Model file for the job. Use its own axes, mm. Face numbers are marked on the shaded views. A direction names the side the tool comes from. Coordinates: 2 decimals unless noted, no trailing zeros. Write each loop counter-clockwise with the first axis right and the second up, starting at its lowest first coordinate (ties: lowest second). Pieces come first, ordered by that corner, then holes. Notation, with made-up numbers: (78.25, 25.25) - (122.25, 25.25) arc R30 cw to (122.25, 53.25) - close; hole circle Ø2 at (54.25, 14.5). An arc over 180 degrees is marked (long way). Put each result on its own line as item: value. Start each with the question number.
1. Saw through at A-A, the plane y = -38.5. Write the cut outline in (x, z).
2. Saw through at C-C, the plane x = -27.5. Write the cut outline in (y, z), plus the area to 3 significant figures.
3. Drill centre lines: L1, parallel to Y at x = -14.5, z = 4.5; L2, parallel to X at y = -35.75, z = 4.5; L3, parallel to X at y = -43.25, z = 4. Where is each one in solid material? Low to high. Write a range as from..to.
4. Drop flat-ended pins along their axis: P1, Ø2, axis at y = -47, z = 6, coming from the -X side; P2, Ø1.5, axis at y = -39, z = 1, coming from the +X side. Give the stop position or say it passes through.
5. Pull direction X, two halves, no side cores. Call the marked faces 4, 5, 6 and 7: released by +X, released by -X, zero draft, split by the parting line, or undercut.
6. Which spindle directions (+Z, -Z, +X, -X, +Y, -Y) get a long thin tool onto all of the face, cutting with end or side? Do the marked faces 1, 2 and 3. Say none if no direction does.
7. Saw through at D-D, the plane z = 6. Write the cut outline in (x, y), plus the area to 3 significant figures.
8. Saw through at B-B, the plane z = 3. Write the cut outline in (x, y), plus the area to 3 significant figures.
```python
from build123d import *

# Parameters (mm, degrees)
F1_DEPTH     = 7
F2_T1_DEPTH  = 32
F2_T3_DEPTH  = 40
F2_T5_DEPTH  = 22
F2_T7_DEPTH  = 11
F2_T10_ANGLE = 90
F2_T12_ANGLE = 90
F2_T14_ANGLE = 90
F2_T16_ANGLE = 90
F2_T18_ANGLE = 90
F2_T20_ANGLE = 90
F2_T22_ANGLE = 90
F2_T24_ANGLE = 90


# Not quite as in the source:
# - a fillet or chamfer that OpenCascade refuses, or shapes differently, is made with other operations: its cross-section is extruded or revolved along the edge and cut away or added


with BuildPart() as f1:
    # F0 (on Top) → F1 (new body)
    with BuildSketch(Plane.XY):
        with BuildLine():
            Line((-4.4512270018, -28.9949133558), (-54.4512270018, -28.9949133558))
            Line((-54.4512270018, -28.9949133558), (-54.4512270018, -45.9949133558))
            ThreePointArc((-54.4512270018, -45.9949133558), (-52.9867609078, -49.5304472618), (-49.4512270018, -50.9949133558))
            Line((-49.4512270018, -50.9949133558), (-9.4512270018, -50.9949133558))
            ThreePointArc((-9.4512270018, -50.9949133558), (-5.9156930959, -49.5304472618), (-4.4512270018, -45.9949133558))
            Line((-4.4512270018, -45.9949133558), (-4.4512270018, -28.9949133558))
        make_face()
        with BuildLine():
            Line((-50.4512270018, -42.9949133558), (-50.4512270018, -31.9949133558))
            Line((-50.4512270018, -31.9949133558), (-8.4512270018, -31.9949133558))
            Line((-8.4512270018, -31.9949133558), (-8.4512270018, -42.9949133558))
            ThreePointArc((-8.4512270018, -42.9949133558), (-9.9156930959, -46.5304472618), (-13.4512270018, -47.9949133558))
            Line((-13.4512270018, -47.9949133558), (-45.4512270018, -47.9949133558))
            ThreePointArc((-45.4512270018, -47.9949133558), (-48.9867609078, -46.5304472618), (-50.4512270018, -42.9949133558))
        make_face(mode=Mode.SUBTRACT)
    extrude(amount=F1_DEPTH)

    # F2: fillet of radius 2 on 4 edges, made by hand

    # F2_s2 → F2_t1 (cut)
    with BuildSketch(Plane.YZ.offset(-45.4512270018)):
        with BuildLine():
            ThreePointArc((-47.9949133558, 5), (-48.5806997934, 6.4142135624), (-49.9949133558, 7))
            Line((-49.9949133558, 7), (-47.9949133558, 7))
            Line((-47.9949133558, 7), (-47.9949133558, 5))
        make_face()
        with BuildLine():
            ThreePointArc((-47.9949133558, 2), (-48.5806997934, 0.5857864376), (-49.9949133558, 0))
            Line((-49.9949133558, 0), (-47.9949133558, 0))
            Line((-47.9949133558, 0), (-47.9949133558, 2))
        make_face()
    extrude(amount=F2_T1_DEPTH, mode=Mode.SUBTRACT)

    # F2_s4 → F2_t3 (cut)
    with BuildSketch(Plane.YZ.offset(-49.4512270018)):
        with BuildLine():
            ThreePointArc((-50.9949133558, 5), (-50.4091269182, 6.4142135624), (-48.9949133558, 7))
            Line((-48.9949133558, 7), (-50.9949133558, 7))
            Line((-50.9949133558, 7), (-50.9949133558, 5))
        make_face()
        with BuildLine():
            ThreePointArc((-50.9949133558, 2), (-50.4091269182, 0.5857864376), (-48.9949133558, 0))
            Line((-48.9949133558, 0), (-50.9949133558, 0))
            Line((-50.9949133558, 0), (-50.9949133558, 2))
        make_face()
    extrude(amount=F2_T3_DEPTH, mode=Mode.SUBTRACT)

    # F2_s6 → F2_t5 (cut)
    with BuildSketch(Plane.XZ.offset(23.9949133558)):
        with BuildLine():
            ThreePointArc((-54.4512270018, 2), (-53.8654405642, 0.5857864376), (-52.4512270018, 0))
            Line((-52.4512270018, 0), (-54.4512270018, 0))
            Line((-54.4512270018, 0), (-54.4512270018, 2))
        make_face()
        with BuildLine():
            ThreePointArc((-4.4512270018, 2), (-5.0370134395, 0.5857864376), (-6.4512270018, 0))
            Line((-6.4512270018, 0), (-4.4512270018, 0))
            Line((-4.4512270018, 0), (-4.4512270018, 2))
        make_face()
        with BuildLine():
            ThreePointArc((-4.4512270018, 5), (-5.0370134395, 6.4142135624), (-6.4512270018, 7))
            Line((-6.4512270018, 7), (-4.4512270018, 7))
            Line((-4.4512270018, 7), (-4.4512270018, 5))
        make_face()
        with BuildLine():
            ThreePointArc((-54.4512270018, 5), (-53.8654405642, 6.4142135624), (-52.4512270018, 7))
            Line((-52.4512270018, 7), (-54.4512270018, 7))
            Line((-54.4512270018, 7), (-54.4512270018, 5))
        make_face()
    extrude(amount=F2_T5_DEPTH, mode=Mode.SUBTRACT)

    # F2_s8 → F2_t7 (cut)
    with BuildSketch(Plane.XZ.offset(31.9949133558)):
        with BuildLine():
            ThreePointArc((-50.4512270018, 2), (-51.0370134395, 0.5857864376), (-52.4512270018, 0))
            Line((-52.4512270018, 0), (-50.4512270018, 0))
            Line((-50.4512270018, 0), (-50.4512270018, 2))
        make_face()
        with BuildLine():
            ThreePointArc((-8.4512270018, 2), (-7.8654405642, 0.5857864376), (-6.4512270018, 0))
            Line((-6.4512270018, 0), (-8.4512270018, 0))
            Line((-8.4512270018, 0), (-8.4512270018, 2))
        make_face()
        with BuildLine():
            ThreePointArc((-50.4512270018, 5), (-51.0370134395, 6.4142135624), (-52.4512270018, 7))
            Line((-52.4512270018, 7), (-50.4512270018, 7))
            Line((-50.4512270018, 7), (-50.4512270018, 5))
        make_face()
        with BuildLine():
            ThreePointArc((-8.4512270018, 5), (-7.8654405642, 6.4142135624), (-6.4512270018, 7))
            Line((-6.4512270018, 7), (-8.4512270018, 7))
            Line((-8.4512270018, 7), (-8.4512270018, 5))
        make_face()
    extrude(amount=F2_T7_DEPTH, mode=Mode.SUBTRACT)

    # F2_s9 → F2_t10 (revolve, cut)
    with BuildSketch(Plane.XZ.offset(42.9949133558)):
        with BuildLine():
            ThreePointArc((-8.4512270018, 2), (-7.8654405642, 0.5857864376), (-6.4512270018, 0))
            Line((-6.4512270018, 0), (-8.4512270018, 0))
            Line((-8.4512270018, 0), (-8.4512270018, 2))
        make_face()
    revolve(axis=Axis((-13.4512270018, -42.9949133558, 0), (0, 0, -1)), revolution_arc=F2_T10_ANGLE, mode=Mode.SUBTRACT)

    # F2_s11 → F2_t12 (revolve, cut)
    with BuildSketch(Plane.YZ.offset(-45.4512270018)):
        with BuildLine():
            ThreePointArc((-47.9949133558, 2), (-48.5806997934, 0.5857864376), (-49.9949133558, 0))
            Line((-49.9949133558, 0), (-47.9949133558, 0))
            Line((-47.9949133558, 0), (-47.9949133558, 2))
        make_face()
    revolve(axis=Axis((-45.4512270018, -42.9949133558, 0), (0, 0, -1)), revolution_arc=F2_T12_ANGLE, mode=Mode.SUBTRACT)

    # F2_s13 → F2_t14 (revolve, cut)
    with BuildSketch(Plane.XZ.offset(45.9949133558)):
        with BuildLine():
            ThreePointArc((-54.4512270018, 2), (-53.8654405642, 0.5857864376), (-52.4512270018, 0))
            Line((-52.4512270018, 0), (-54.4512270018, 0))
            Line((-54.4512270018, 0), (-54.4512270018, 2))
        make_face()
    revolve(axis=Axis((-49.4512270018, -45.9949133558, 0), (0, 0, 1)), revolution_arc=F2_T14_ANGLE, mode=Mode.SUBTRACT)

    # F2_s15 → F2_t16 (revolve, cut)
    with BuildSketch(Plane.YZ.offset(-9.4512270018)):
        with BuildLine():
            ThreePointArc((-50.9949133558, 2), (-50.4091269182, 0.5857864376), (-48.9949133558, 0))
            Line((-48.9949133558, 0), (-50.9949133558, 0))
            Line((-50.9949133558, 0), (-50.9949133558, 2))
        make_face()
    revolve(axis=Axis((-9.4512270018, -45.9949133558, 0), (0, 0, 1)), revolution_arc=F2_T16_ANGLE, mode=Mode.SUBTRACT)

    # F2_s17 → F2_t18 (revolve, cut)
    with BuildSketch(Plane.XZ.offset(45.9949133558)):
        with BuildLine():
            ThreePointArc((-54.4512270018, 5), (-53.8654405642, 6.4142135624), (-52.4512270018, 7))
            Line((-52.4512270018, 7), (-54.4512270018, 7))
            Line((-54.4512270018, 7), (-54.4512270018, 5))
        make_face()
    revolve(axis=Axis((-49.4512270018, -45.9949133558, 7), (0, 0, 1)), revolution_arc=F2_T18_ANGLE, mode=Mode.SUBTRACT)

    # F2_s19 → F2_t20 (revolve, cut)
    with BuildSketch(Plane.YZ.offset(-9.4512270018)):
        with BuildLine():
            ThreePointArc((-50.9949133558, 5), (-50.4091269182, 6.4142135624), (-48.9949133558, 7))
            Line((-48.9949133558, 7), (-50.9949133558, 7))
            Line((-50.9949133558, 7), (-50.9949133558, 5))
        make_face()
    revolve(axis=Axis((-9.4512270018, -45.9949133558, 7), (0, 0, 1)), revolution_arc=F2_T20_ANGLE, mode=Mode.SUBTRACT)

    # F2_s21 → F2_t22 (revolve, cut)
    with BuildSketch(Plane.XZ.offset(42.9949133558)):
        with BuildLine():
            ThreePointArc((-8.4512270018, 5), (-7.8654405642, 6.4142135624), (-6.4512270018, 7))
            Line((-6.4512270018, 7), (-8.4512270018, 7))
            Line((-8.4512270018, 7), (-8.4512270018, 5))
        make_face()
    revolve(axis=Axis((-13.4512270018, -42.9949133558, 7), (0, 0, -1)), revolution_arc=F2_T22_ANGLE, mode=Mode.SUBTRACT)

    # F2_s23 → F2_t24 (revolve, cut)
    with BuildSketch(Plane.YZ.offset(-45.4512270018)):
        with BuildLine():
            ThreePointArc((-47.9949133558, 5), (-48.5806997934, 6.4142135624), (-49.9949133558, 7))
            Line((-49.9949133558, 7), (-47.9949133558, 7))
            Line((-47.9949133558, 7), (-47.9949133558, 5))
        make_face()
    revolve(axis=Axis((-45.4512270018, -42.9949133558, 7), (0, 0, -1)), revolution_arc=F2_T24_ANGLE, mode=Mode.SUBTRACT)


solid = f1.part
```
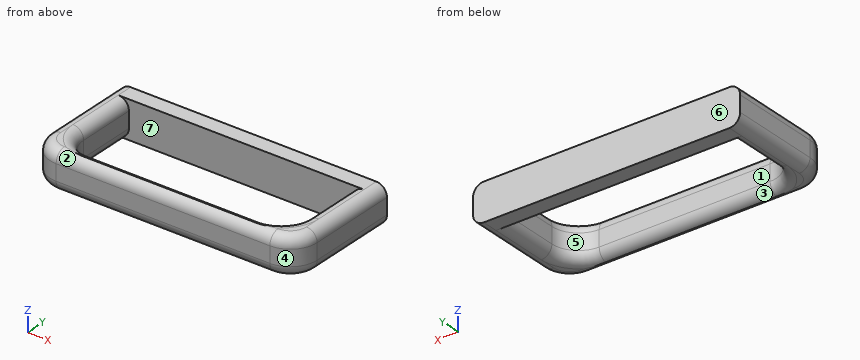
Final values:
1. outline: (-54.45, 2) arc R2 ccw to (-50.45, 2) - (-50.45, 5) arc R2 ccw to (-54.45, 5) - close; (-8.45, 2) arc R2 ccw to (-4.45, 2) - (-4.45, 5) arc R2 ccw to (-8.45, 5) - close
2. outline: (-50.99, 2) arc R2 ccw to (-49.49, 0.06) arc R2 ccw to (-47.99, 2) - (-47.99, 5) arc R2 ccw to (-49.49, 6.94) arc R2 ccw to (-50.99, 5) - close; (-31.99, 0) - (-28.99, 0) - (-28.99, 7) - (-31.99, 7) - close
2. area: 38.6 mm²
3. L1: y = -50.99..-47.99, -31.99..-28.99
3. L2: x = -54.45..-50.45, -8.45..-4.45
3. L3: x = -54.45..-50.44, -8.46..-4.45
4. P1: stops at x = -54.42
4. P2: stops at x = -4.47
5. face 4: released by +X
5. face 5: undercut
5. face 6: zero draft
5. face 7: undercut
6. face 1: +Z, -Z
6. face 2: +Z, +X, -X, -Y
6. face 3: -Z
7. outline: (-54.18, -45.99) arc R4.73 ccw to (-49.45, -50.73) - (-9.45, -50.73) arc R4.73 ccw to (-4.72, -45.99) - (-4.72, -28.99) - (-54.18, -28.99) - close; hole (-50.72, -42.99) arc R5.27 ccw to (-45.45, -48.26) - (-13.45, -48.26) arc R5.27 ccw to (-8.18, -42.99) - (-8.18, -31.99) - (-50.72, -31.99) - close
7. area: 385 mm²
8. outline: (-54.45, -45.99) arc R5 ccw to (-49.45, -50.99) - (-9.45, -50.99) arc R5 ccw to (-4.45, -45.99) - (-4.45, -28.99) - (-54.45, -28.99) - close; hole (-50.45, -42.99) arc R5 ccw to (-45.45, -47.99) - (-13.45, -47.99) arc R5 ccw to (-8.45, -42.99) - (-8.45, -31.99) - (-50.45, -31.99) - close
8. area: 428 mm²
